Verification items for this drawing (mm, ordinates from the low corner). Give positions to 0.01 mm unless a question says otherwise; leave off trailing zeros. Loops run counter-clockwise (first coordinate to the right, second up) from the corner with the lowest first, then second, coordinate; pieces in that order, holes last. Notation, with made-up numbers: M 2.5,9.25 L 60.5,9.25 A30 cw 60.5,33.25 Z; hole C 32,24 d2. An arc over 180 degrees is marked long. Use one line per item in the form item = value.
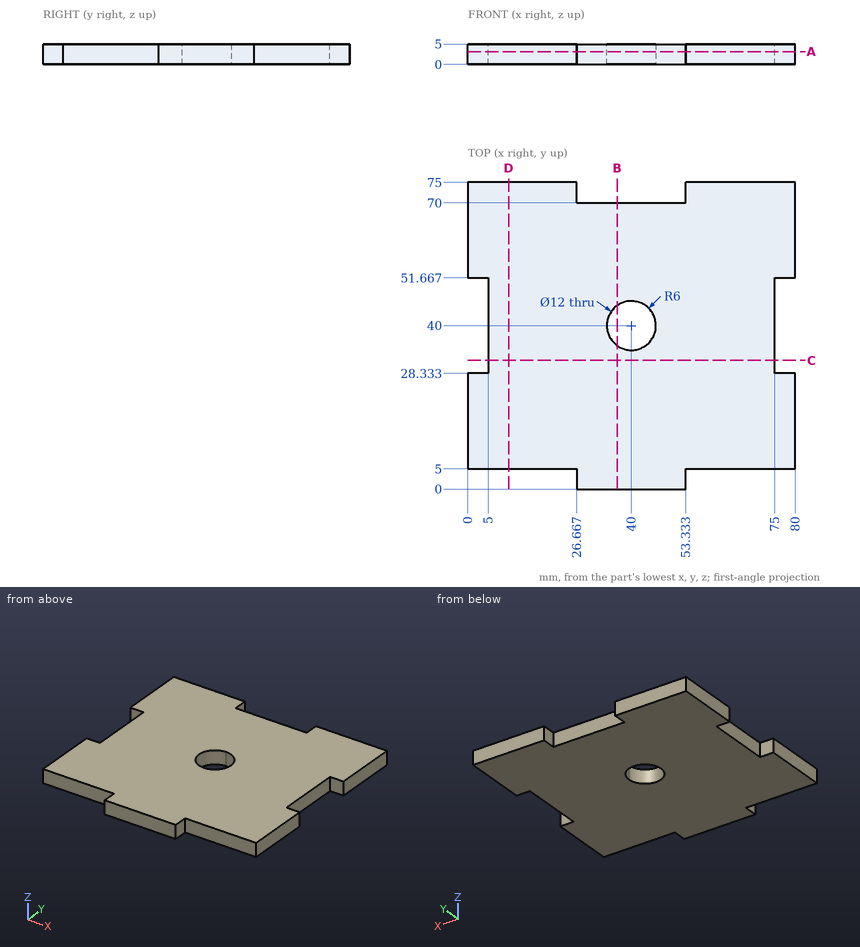
1) Section check C-C (y = 31.5). Record the cut outline in (x, z), then the cut area to 3 significant figures.
Evaluation:
outline = M 5,0 L 75,0 L 75,5 L 5,5 Z
area = 350 mm^2
2) Section check B-B (x = 36.5). Record the cut outline in (y, z), then the cut area to 3 significant figures.
Evaluation:
outline = M 0,0 L 35.13,0 L 35.13,5 L 0,5 Z; M 44.87,0 L 70,0 L 70,5 L 44.87,5 Z
area = 301 mm^2
3) Depth check by flat-ended pin: pin 1 Ø2.5 at (y, z) = (36.5, 3) entering from +X; pin 2 Ø1.5 at (x, z) = (69, 1.5) entering from -Y; pin 3 Ø3 at (y, z) = (59.5, 3) entering from -X; pin 4 Ø2.5 at (y, z) = (1.5, 2.5) entering from +X. Enter the tip coordinate at first touch or a pass-through.
Evaluation:
pin_1 = 75
pin_2 = 5
pin_3 = 0
pin_4 = 53.33
4) Section check A-A (z = 3.15). Record the cut outline in (x, y), then the cut area to 3 significant figures.
Evaluation:
outline = M 0,5 L 26.67,5 L 26.67,0 L 53.33,0 L 53.33,5 L 80,5 L 80,28.33 L 75,28.33 L 75,51.67 L 80,51.67 L 80,75 L 53.33,75 L 53.33,70 L 26.67,70 L 26.67,75 L 0,75 L 0,51.67 L 5,51.67 L 5,28.33 L 0,28.33 Z; hole C 40,40 d12
area = 5,250 mm^2
5) Scan lines: line 1 (X direction, y = 40, z = 1.15); line 2 (Y direction, x = 40, z = 1.25); line 3 (Y direction, x = 25.5, z = 2.85). Record each from-to range of solid material in increasing order.
Evaluation:
line_1 = 5 to 34, 46 to 75
line_2 = 0 to 34, 46 to 70
line_3 = 5 to 75
